Part model, mm, in its own coordinate system. Face numbers are marked on the shaded views. A direction names the side the tool comes from. Give positions to 0.01 mm unless a question says otherwise; leave off trailing zeros. Write each loop counter-clockwise with the first axis right and the second up, starting at its lowest first coordinate (ties: lowest second). Pieces come first, ordered by that corner, then holes.
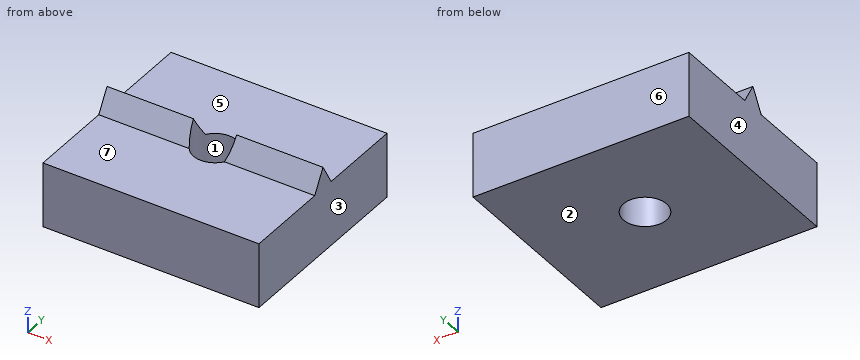
from build123d import *

# Parameters (mm, degrees)
SKETCH1_W           = 10
SKETCH1_H           = 9
BOSS_EXTRUDE1_DEPTH = 3
BOSS_EXTRUDE2_DEPTH = 10
CUT_EXTRUDE1_REACH  = 9.826
SKETCH3_R           = 1


with BuildPart() as part:
    # Sketch1 → Boss-Extrude1 (new body)
    with BuildSketch(Plane.XY):
        Rectangle(SKETCH1_W, SKETCH1_H)
    extrude(amount=BOSS_EXTRUDE1_DEPTH)

    # Sketch2 → Boss-Extrude2 (add)
    with BuildSketch(Plane(origin=(5, 0, 0), x_dir=(0, 0, -1), z_dir=(1, 0, 0))):
        Polygon((-4, 0), (-2.5, -0.866025404), (-2.5, 0.866025404), align=None)
    extrude(amount=-BOSS_EXTRUDE2_DEPTH)

    # Sketch3 → Cut-Extrude1 (cut, up to next)
    with BuildSketch(Plane(origin=(0, 0, 0), x_dir=(-1, 0, 0), z_dir=(0, 0, -1)), mode=Mode.PRIVATE) as cut_extrude1_sk1:
        Circle(SKETCH3_R)
    cut_extrude1_tool1 = extrude(cut_extrude1_sk1.sketch, amount=-CUT_EXTRUDE1_REACH, mode=Mode.PRIVATE) & part.part
    add(cut_extrude1_tool1.solids().sort_by_distance((0, 0, 0))[0], mode=Mode.SUBTRACT)


solid = part.part
1) Mould opens along X. For the marked faces 1, 2, 3 and 4 say: +X half, -X half, draft (parallel to the pull), parting line (faces both ways), or undercut.
Check result:
face 1: undercut
face 2: draft
face 3: +X half
face 4: -X half
2) Saw through at C-C (x = -4). Write the cut outline in (y, z), and give its area (3 significant figures).
Check result:
outline: (-4.5, 0) - (4.5, 0) - (4.5, 3) - (0.58, 3) - (0, 4) - (-0.58, 3) - (-4.5, 3) - close
area: 27.6 mm2
3) Saw through at B-B (z = 0.6). Write the cut outline in (x, y).
Check result:
outline: (-5, -4.5) - (5, -4.5) - (5, 4.5) - (-5, 4.5) - close; hole circle Ø2 at (0, 0)
4) 3-axis set-ups, long thin cutter, end or side, ignore diameter. For the marked faces 5, 6 and 7: which of +Z, -Z, +X, -X, +Y, -Y reach the whole face in a straight line?
Check result:
face 5: +Z, +X, -X, +Y
face 6: +Z, -Z, +X, -X, +Y
face 7: +Z, +X, -X, -Y
5) Saw through at A-A (x = 0). Write the cut outline in (y, z), and give its area (3 significant figures).
Check result:
outline: (-4.5, 0) - (-1, 0) - (-1, 3) - (-4.5, 3) - close; (1, 0) - (4.5, 0) - (4.5, 3) - (1, 3) - close
area: 21.0 mm2
6) Drill centre lines: L1, parallel to Y at x = 0, z = 2.1; L2, parallel to X at y = 0, z = 3.4; L3, parallel to Z at x = 4.5, y = -3.75. Where is each one in solid material? Low to high.
Check result:
L1: y = -4.5 to -1, 1 to 4.5
L2: x = -5 to -1, 1 to 5
L3: z = 0 to 3
7) Flat gauge pins, fed straight in: P1, Ø2, axis at x = -0.5, y = -2.5, coming from the +Z side; P2, Ø1, axis at x = 4, y = 1, coming from the +Z side. Where does each tip first touch, or does it go through?
Check result:
P1: stops at z = 3
P2: stops at z = 3.13
8) Saw through at D-D (y = 0.25). Write the cut outline in (x, z).
Check result:
outline: (-5, 0) - (-0.97, 0) - (-0.97, 3.57) - (-5, 3.57) - close; (0.97, 0) - (5, 0) - (5, 3.57) - (0.97, 3.57) - close
